Check sheet for the modelled part. Datum: model origin and axes. Units: mm. Coordinates: 2 decimals unless noted, no trailing zeros. Write each loop counter-clockwise with the first axis right and the second up, starting at its lowest first coordinate (ties: lowest second). Pieces come first, ordered by that corner, then holes. Notation, with made-up numbers: M 71.25,26 L 120.25,26 A26 ccw 120.25,51 Z; hole C -14.75,-28 d5. An arc over 180 degrees is marked long. Answer as CSV lines item,"result".
from build123d import *

# Parameters (mm, degrees)
F0_W     = 40
F0_H     = 1875
F0_R     = 6
F1_DEPTH = 40
F2_W     = 32
F2_H     = 32
F3_DEPTH = 1875.001


with BuildPart() as f1:
    # F0 (on Front) → F1 (new body)
    with BuildSketch(Plane.XZ):
        with Locations((20, 927.753484)):
            Rectangle(F0_W, F0_H)
        with Locations((20, 15.253484)):
            Circle(F0_R, mode=Mode.SUBTRACT)
        with Locations((20, 1840.253484)):
            Circle(F0_R, mode=Mode.SUBTRACT)
    extrude(amount=F1_DEPTH)

    # F2 (on face) → F3 (cut, through all)
    with BuildSketch(Plane.XY.offset(1865.253484)):
        with Locations((20, -20)):
            Rectangle(F2_W, F2_H)
    extrude(amount=-F3_DEPTH, mode=Mode.SUBTRACT)


solid = f1.part
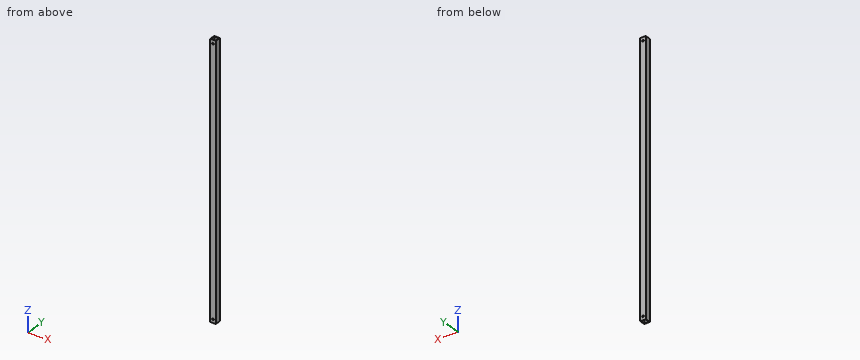
1) Section check B-B, the plane z = 1430. Record the boundary of the cut face in (x, y).
Answer key:
outline,"M 0,-40 L 40,-40 L 40,0 L 0,0 Z; hole M 4,-36 L 36,-36 L 36,-4 L 4,-4 Z"
2) Depth check by flat-ended pin: P1, Ø1, axis at x = 5, y = -12.5, coming from the -Z side. Enter the tip coordinate at first touch or a pass-through.
Answer key:
P1,"passes through"
3) Thickness scan on line 1 along Z through (x, y) = (20, -2.1); line 2 along Y through (x, z) = (28, 469); line 3 along X through (y, z) = (-31, 667). Record the ranges inside material, lowest first.
Answer key:
line 1,"z = -9.75 to 9.25, 21.25 to 1834.25, 1846.25 to 1865.25"
line 2,"y = -40 to -36, -4 to 0"
line 3,"x = 0 to 4, 36 to 40"
4) Section check A-A, the plane x = 20. Record the boundary of the cut face in (y, z), plus the area to 3 significant figures.
Answer key:
outline,"M -40,-9.75 L -36,-9.75 L -36,9.25 L -40,9.25 Z; M -40,21.25 L -36,21.25 L -36,1834.25 L -40,1834.25 Z; M -40,1846.25 L -36,1846.25 L -36,1865.25 L -40,1865.25 Z; M -4,-9.75 L 0,-9.75 L 0,9.25 L -4,9.25 Z; M -4,21.25 L 0,21.25 L 0,1834.25 L -4,1834.25 Z; M -4,1846.25 L 0,1846.25 L 0,1865.25 L -4,1865.25 Z"
area,"14,800 mm2"
